The model under review builds one solid part; all positions refer to its coordinate system, in mm. Round coordinates to 2 decimals unless told otherwise and drop trailing zeros. Order: outer loops, then holes, each group sorted by start corner. A loop starts at its lowest first (then second) coordinate and runs counter-clockwise, first axis right, second up. Notation, with made-up numbers: (9.25, 67) -> (49.25, 67) arc R16 cw to (49.25, 76) -> close; hole circle Ø10 at (-37.5, 64). An arc over 180 degrees is marked (long way). Return JSON: item names as keys, results as strings. Group by question number.
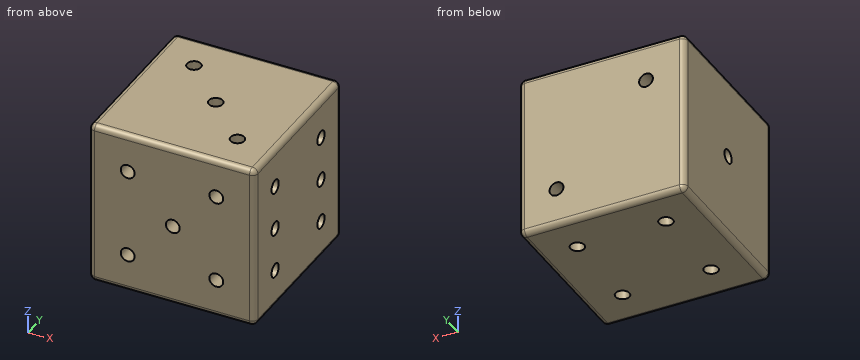
from build123d import *

# Parameters (mm, degrees)
F1_DEPTH     = 15
F2_R         = 1
F3_T1_DEPTH  = 28
F3_S5_W      = 1
F3_S5_H      = 1
F3_T6_DEPTH  = 1
F3_S11_W     = 1
F3_S11_H     = 1
F3_T12_DEPTH = 1
F10_D        = 2.5
F10_DEPTH    = 3
F10_TIP      = 0.7510757738
F11_D        = 2.5
F11_DEPTH    = 3
F11_TIP      = 0.7510757738
F12_D        = 2.5
F12_DEPTH    = 3
F12_TIP      = 0.7510757738
F13_D        = 2.5
F13_DEPTH    = 3
F13_TIP      = 0.7510757738
F14_D        = 2.5
F14_DEPTH    = 3
F14_TIP      = 0.7510757738
F15_D        = 2.5
F15_DEPTH    = 3
F15_TIP      = 0.7510757738


# Not quite as in the source:
# - a fillet or chamfer that OpenCascade refuses, or shapes differently, is made with other operations: its cross-section is extruded or revolved along the edge and cut away or added


with BuildPart() as f1:
    # F0 (on Front) → F1 (new body, symmetric)
    with BuildSketch(Plane.XZ):
        Polygon((-0.1339098811, 0.0507837534), (-15.1339098811, 15.0507837534), (-15.1339098811, -14.9492162466), align=None)
        Polygon((14.8660901189, 15.0507837534), (-15.1339098811, 15.0507837534), (-0.1339098811, 0.0507837534), align=None)
        Polygon((14.8660901189, -14.9492162466), (14.8660901189, 15.0507837534), (-0.1339098811, 0.0507837534), align=None)
        Polygon((-0.1339098811, 0.0507837534), (-15.1339098811, -14.9492162466), (14.8660901189, -14.9492162466), align=None)
    extrude(amount=F1_DEPTH, both=True)

    # F2
    f2_edges = [f1.edges().sort_by_distance(p)[0] for p in [
        (-0.13391, -15, 15.050784),
        (14.86609, 0, 15.050784),
        (-0.13391, 15, 15.050784),
        (-15.13391, 0, 15.050784),
        (-15.13391, 15, 0.050784),
        (14.86609, 15, 0.050784),
        (14.86609, -15, 0.050784),
        (-0.13391, -15, -14.949216),
        (14.86609, 0, -14.949216),
        (-15.13391, 0, -14.949216),
        (-0.13391, 15, -14.949216),
    ]]
    fillet(f2_edges, radius=F2_R)

    # F3: fillet of radius 1 on 1 edges, made by hand

    # F3_s2 → F3_t1 (cut)
    with BuildSketch(Plane.XY.offset(-13.9492162466)):
        with BuildLine():
            ThreePointArc((-15.1339098811, -14), (-14.8410166623, -14.7071067812), (-14.1339098811, -15))
            Line((-14.1339098811, -15), (-15.1339098811, -15))
            Line((-15.1339098811, -15), (-15.1339098811, -14))
        make_face()
    extrude(amount=F3_T1_DEPTH, mode=Mode.SUBTRACT)


with BuildPart() as f3_tool4:
    # F3_s5 → F3_t6 (new body)
    with BuildSketch(Plane.YZ.offset(-14.1339098811)):
        with Locations((-14.5, 14.5507837534)):
            Rectangle(F3_S5_W, F3_S5_H)
    extrude(amount=-F3_T6_DEPTH)

    # F3_s7 → F3_t8 (revolve, cut)
    with BuildSketch(Plane(origin=(-14.1339098811, -14, 14.0507837534), x_dir=(0, 0.7071067812, -0.7071067812), z_dir=(0, 0.7071067812, 0.7071067812))):
        with BuildLine():
            ThreePointArc((0, -1), (1, 0), (0, 1))
            Line((0, 1), (0, -1))
        make_face()
    revolve(axis=Axis((-14.1339098811, -14, 14.0507837534), (-1, 0, 0)), mode=Mode.SUBTRACT)


with BuildPart() as f1_1:
    add(f1.part)

    # F3_t3: cut F3_tool4
    add(f3_tool4.part, mode=Mode.SUBTRACT)


with BuildPart() as f3_tool10:
    # F3_s11 → F3_t12 (new body)
    with BuildSketch(Plane.YZ.offset(-14.1339098811)):
        with Locations((-14.5, -14.4492162466)):
            Rectangle(F3_S11_W, F3_S11_H)
    extrude(amount=-F3_T12_DEPTH)

    # F3_s13 → F3_t14 (revolve, cut)
    with BuildSketch(Plane(origin=(-14.1339098811, -14, -13.9492162466), x_dir=(0, 0.7071067812, 0.7071067812), z_dir=(0, -0.7071067812, 0.7071067812))):
        with BuildLine():
            ThreePointArc((0, -1), (1, 0), (0, 1))
            Line((0, 1), (0, -1))
        make_face()
    revolve(axis=Axis((-14.1339098811, -14, -13.9492162466), (-1, 0, 0)), mode=Mode.SUBTRACT)


with BuildPart() as f1_2:
    add(f1_1.part)

    # F3_t9: cut F3_tool10
    add(f3_tool10.part, mode=Mode.SUBTRACT)

    # F10
    with Locations(Plane(origin=(-15.1339098811, 0, 0), x_dir=(0, -1, 0), z_dir=(-1, 0, 0))):
        with Locations((0, 0)):
            Hole(F10_D / 2, depth=F10_DEPTH)
            with Locations((0, 0, -(F10_DEPTH + F10_TIP / 2))):  # 118° drill point
                Cone(0, F10_D / 2, F10_TIP, mode=Mode.SUBTRACT)

    # F11
    with Locations(Plane(origin=(0, 15, 0), x_dir=(-1, 0, 0), z_dir=(0, 1, 0))):
        with Locations((8.0831261277, 8), (-8.0831261277, -8)):
            Hole(F11_D / 2, depth=F11_DEPTH)
            with Locations((0, 0, -(F11_DEPTH + F11_TIP / 2))):  # 118° drill point
                Cone(0, F11_D / 2, F11_TIP, mode=Mode.SUBTRACT)

    # F12
    with Locations(Plane.XY.offset(15.0507837534)):
        with Locations((-8, 7.8672532922), (0, 0), (8, -7.8672532922)):
            Hole(F12_D / 2, depth=F12_DEPTH)
            with Locations((0, 0, -(F12_DEPTH + F12_TIP / 2))):  # 118° drill point
                Cone(0, F12_D / 2, F12_TIP, mode=Mode.SUBTRACT)

    # F13
    with Locations(Plane(origin=(0, 0, -14.9492162466), x_dir=(1, 0, 0), z_dir=(0, 0, -1))):
        with Locations((-8, 7.8660901189), (8, 7.8660901189), (8, -7.8660901189), (-8, -7.8660901189)):
            Hole(F13_D / 2, depth=F13_DEPTH)
            with Locations((0, 0, -(F13_DEPTH + F13_TIP / 2))):  # 118° drill point
                Cone(0, F13_D / 2, F13_TIP, mode=Mode.SUBTRACT)

    # F14
    with Locations(Plane.YZ.offset(14.8660901189)):
        with Locations((-8, 8.0507837534), (-8, 0), (-8, -8.0507837534), (8, -8.0507837534), (8, 0), (8, 8.0507837534)):
            Hole(F14_D / 2, depth=F14_DEPTH)
            with Locations((0, 0, -(F14_DEPTH + F14_TIP / 2))):  # 118° drill point
                Cone(0, F14_D / 2, F14_TIP, mode=Mode.SUBTRACT)

    # F15
    with Locations(Plane.XZ.offset(15)):
        with Locations((-8.1339098811, 8.0507837534), (0, 0), (7.8660901189, 8.0507837534), (7.8660901189, -7.9492162466), (-8.1339098811, -7.9492162466)):
            Hole(F15_D / 2, depth=F15_DEPTH)
            with Locations((0, 0, -(F15_DEPTH + F15_TIP / 2))):  # 118° drill point
                Cone(0, F15_D / 2, F15_TIP, mode=Mode.SUBTRACT)


solid = f1_2.part
Item 1: Consider section A-A on x = 12.75. State the section outline as (y, z) points.
Item 2: Wall thickness on line 1 along Y through (x, z) = (8, -12.9); line 2 along Y through (x, z) = (13, 0); line 3 along Z through (x, y) = (14.1, 8): over which ranges is each line inside the solid? List them lowest first.
Item 3: Insertion check: pin 1 Ø2 at (y, z) = (-8, 8.05) entering from +X; pin 2 Ø2 at (x, z) = (8.08, -8) entering from -Y; pin 3 Ø1.5 at (x, y) = (-8, 7.87) entering from +Z. Each pin has a flat end and moves straight along its axis. Give the tip position at first contact, or say it passes through.
Values:
{
 "1": {"outline": "(-15, -13.95) arc R1 ccw to (-14, -14.95) -> (14, -14.95) arc R1 ccw to (15, -13.95) -> (15, 14.05) arc R1 ccw to (14, 15.05) -> (-14, 15.05) arc R1 ccw to (-15, 14.05) -> close; hole circle Ø2.5 at (-8, -8.05); hole circle Ø2.5 at (-8, 0); hole circle Ø2.5 at (-8, 8.05); hole circle Ø2.5 at (8, -8.05); hole circle Ø2.5 at (8, 0); hole circle Ø2.5 at (8, 8.05)"},
 "2": {"line 1": "-15 to -9.12, -6.62 to 6.62, 9.12 to 15", "line 2": "-15 to -9.25, -6.75 to 6.75, 9.25 to 15", "line 3": "-14.92 to -9.3, -6.8 to -1.25, 1.25 to 6.8, 9.3 to 15.02"},
 "3": {"pin 1": "x = 11.72", "pin 2": "y = -11.98", "pin 3": "z = 11.75"}
}
